from build123d import *

# Parameters (mm, degrees)
SKETCH_W     = 31.75
SKETCH_H     = 31.75
SKETCH_W_2   = 26.2128
SKETCH_H_2   = 26.2128
PAD_DEPTH    = 152.4
POCKET_DEPTH = 31.75


with BuildPart() as part:
    # Sketch → Pad (new body)
    with BuildSketch(Plane.XY):
        Rectangle(SKETCH_W, SKETCH_H)
        Rectangle(SKETCH_W_2, SKETCH_H_2, mode=Mode.SUBTRACT)
    extrude(amount=PAD_DEPTH)

    # Sketch001 → Pocket (cut)
    with BuildSketch(Plane.YZ.offset(15.875)):
        Polygon((-15.875, 152.4), (15.875, 152.4), (15.875, 120.65), align=None)
    extrude(amount=-POCKET_DEPTH, mode=Mode.SUBTRACT)


solid = part.part
Verification items for the finished model (mm, model axes). A direction names the side the tool comes from. Coordinates: 2 decimals unless noted, no trailing zeros. Loops run counter-clockwise (first coordinate to the right, second up) from the corner with the lowest first, then second, coordinate; pieces in that order, holes last. Notation, with made-up numbers: (-23, -1) -> (0, -1) arc R33 cw to (0, 32) -> close; hole circle Ø10 at (-22.75, 88.5). An arc over 180 degrees is marked (long way). Answer as a JSON object with one key per item and string values. Group by question number.
Item 1: Sectioned sample at C-C on z = 48.5. Record the boundary of the cut face in (x, y) (3 decimals), plus the area to 3 significant figures.
Item 2: Mould release check, pull along X, two halves, no side actions. Record for faces 1 (the flat face through (-13.106, 0, 74)), 2 (the flat face through (-15.875, 0, 75)), 3 (the flat face through (-13.889, 0.222, 136.303)): +X half, -X half, draft (parallel to the pull), parting line (faces both ways), or undercut.
Item 3: Sectioned sample at A-A on x = -1. Record the boundary of the cut face in (y, z) (3 decimals).
Item 4: Tool access check on faces 4 (the flat face through (0, -15.875, 75)), 5 (the flat face through (13.106, 0, 74)). Record the directions out of +Z, -Z, +X, -X, +Y, -Y that give a thin tool (end or side, any length) a straight path to the whole face; none if there is none.
Item 5: Scan lines: probe 1 along Y at (x, z) = (-8.5, 33.5) (3 decimals); probe 2 along Y at (x, z) = (-10.5, 122) (3 decimals). Record each from-to range of solid material in increasing order.
Item 6: Sectioned sample at B-B on y = 0. Record the boundary of the cut face in (x, z) (3 decimals).
Item 7: Sectioned sample at D-D on z = 128.5. Record the boundary of the cut face in (x, y) (3 decimals).
Evaluation:
{
 "1": {"outline": "(-15.875, -15.875) -> (15.875, -15.875) -> (15.875, 15.875) -> (-15.875, 15.875) -> close; hole (-13.106, -13.106) -> (13.106, -13.106) -> (13.106, 13.106) -> (-13.106, 13.106) -> close", "area": "321 mm²"},
 "2": {"face 1": "undercut", "face 2": "-X half", "face 3": "draft"},
 "3": {"outline": "(-15.875, 0) -> (-13.106, 0) -> (-13.106, 149.631) -> (-15.875, 152.4) -> close; (13.106, 0) -> (15.875, 0) -> (15.875, 120.65) -> (13.106, 123.419) -> close"},
 "4": {"face 4": "+Z, -Z, +X, -X, -Y", "face 5": "+Z, -Z"},
 "5": {"probe 1": "y = -15.875 to -13.106, 13.106 to 15.875", "probe 2": "y = -15.875 to -13.106, 13.106 to 14.525"},
 "6": {"outline": "(-15.875, 0) -> (-13.106, 0) -> (-13.106, 136.525) -> (-15.875, 136.525) -> close; (13.106, 0) -> (15.875, 0) -> (15.875, 136.525) -> (13.106, 136.525) -> close"},
 "7": {"outline": "(-15.875, -15.875) -> (15.875, -15.875) -> (15.875, 8.025) -> (13.106, 8.025) -> (13.106, -13.106) -> (-13.106, -13.106) -> (-13.106, 8.025) -> (-15.875, 8.025) -> close"}
}
